```python
from build123d import *

# Parameters (mm, degrees)
SKETCH1_R               = 43
SKETCH1_R_2             = 9.5
SKETCH1_R_3             = 3
BOSS_EXTRUDE1_DEPTH     = 6
CUT_EXTRUDE1_DEPTH      = 62.983868869
CUT_EXTRUDE1_DEPTH_BACK = 62.983868869


with BuildPart() as part:
    # Sketch1 → Boss-Extrude1 (new, symmetric)
    with BuildSketch(Plane(origin=(0, 0, 0), x_dir=(1, 0, 0), z_dir=(0, 1, 0))):
        with Locations(Location((0, 0, 0), (0, 0, 270))):
            Circle(SKETCH1_R)
        with Locations(Location((0, 0, 0), (0, 0, 270))):
            Circle(SKETCH1_R_2, mode=Mode.SUBTRACT)
        with Locations(Location((0, -32, 0), (0, 0, 270))):
            Circle(SKETCH1_R_3, mode=Mode.SUBTRACT)
        with Locations(Location((-30.433808521, -9.88854382, 0), (0, 0, 270))):
            Circle(SKETCH1_R_3, mode=Mode.SUBTRACT)
        with Locations(Location((-18.809128073, 25.88854382, 0), (0, 0, 270))):
            Circle(SKETCH1_R_3, mode=Mode.SUBTRACT)
        with Locations(Location((18.809128073, 25.88854382, 0), (0, 0, 270))):
            Circle(SKETCH1_R_3, mode=Mode.SUBTRACT)
        with Locations(Location((30.433808521, -9.88854382, 0), (0, 0, 270))):
            Circle(SKETCH1_R_3, mode=Mode.SUBTRACT)
    extrude(amount=BOSS_EXTRUDE1_DEPTH, both=True)

    # Sketch2 → Cut-Extrude1 (cut, two sides: drawn at the far end of the back side and taken through both)
    with BuildSketch(Plane(origin=(0, 6, 0), x_dir=(1, 0, 0), z_dir=(0, 1, 0)).offset(-CUT_EXTRUDE1_DEPTH_BACK)):
        with BuildLine():
            ThreePointArc((-9.114016839, 9.270096928), (-12.363734712, 4.017220927), (-12.822220771, -2.142581267))
            ThreePointArc((-12.822220771, -2.142581267), (-21.270303496, -1.833512485), (-29.494654795, 0.122419764))
            ThreePointArc((-29.494654795, 0.122419764), (-32.446074444, 2.845461233), (-32.44271131, 6.861158119))
            ThreePointArc((-32.44271131, 6.861158119), (-31.194730701, 10.135782424), (-30.27959235, 13.518553733))
            ThreePointArc((-30.27959235, 13.518553733), (-27.921945775, 16.769297559), (-23.933633504, 17.23748344))
            ThreePointArc((-23.933633504, 17.23748344), (-16.130325405, 13.985713467), (-9.114016839, 9.270096928))
        make_face()
        with BuildLine():
            ThreePointArc((6, 11.532562595), (0, 13), (-6, 11.532562595))
            ThreePointArc((-6, 11.532562595), (-8.316659253, 19.662674227), (-8.99792146, 28.088913426))
            ThreePointArc((-8.99792146, 28.088913426), (-7.320193957, 31.737346406), (-3.5, 32.975066458))
            ThreePointArc((-3.5, 32.975066458), (0, 32.800080928), (3.5, 32.975066458))
            ThreePointArc((3.5, 32.975066458), (7.320193957, 31.737346406), (8.99792146, 28.088913426))
            ThreePointArc((8.99792146, 28.088913426), (8.316659253, 19.662674227), (6, 11.532562595))
        make_face()
        with BuildLine():
            ThreePointArc((12.822220771, -2.142581267), (12.363734712, 4.017220927), (9.114016839, 9.270096928))
            ThreePointArc((9.114016839, 9.270096928), (16.130325405, 13.985713467), (23.933633504, 17.23748344))
            ThreePointArc((23.933633504, 17.23748344), (27.921945775, 16.769297559), (30.27959235, 13.518553733))
            ThreePointArc((30.27959235, 13.518553733), (31.194730701, 10.135782424), (32.44271131, 6.861158119))
            ThreePointArc((32.44271131, 6.861158119), (32.446074444, 2.845461233), (29.494654795, 0.122419764))
            ThreePointArc((29.494654795, 0.122419764), (21.270303496, -1.833512485), (12.822220771, -2.142581267))
        make_face()
        with BuildLine():
            ThreePointArc((-1.924568248, -12.856750642), (-4.829111259, -20.795847261), (-9.230777689, -28.013253851))
            ThreePointArc((-9.230777689, -28.013253851), (-12.732582852, -29.978754651), (-16.550698277, -28.734637538))
            ThreePointArc((-16.550698277, -28.734637538), (-19.279403843, -26.535822888), (-22.213817238, -24.620140772))
            ThreePointArc((-22.213817238, -24.620140772), (-24.576905478, -21.373350548), (-23.78972044, -17.435562779))
            ThreePointArc((-23.78972044, -17.435562779), (-18.285748603, -11.019027947), (-11.632772181, -5.803327614))
            ThreePointArc((-11.632772181, -5.803327614), (-7.64120828, -10.517220927), (-1.924568248, -12.856750642))
        make_face()
        with BuildLine():
            ThreePointArc((1.924568248, -12.856750642), (7.64120828, -10.517220927), (11.632772181, -5.803327614))
            ThreePointArc((11.632772181, -5.803327614), (18.285748603, -11.019027947), (23.78972044, -17.435562779))
            ThreePointArc((23.78972044, -17.435562779), (24.576905478, -21.373350548), (22.213817238, -24.620140772))
            ThreePointArc((22.213817238, -24.620140772), (19.279403843, -26.535822888), (16.550698277, -28.734637538))
            ThreePointArc((16.550698277, -28.734637538), (12.732582852, -29.978754651), (9.230777689, -28.013253851))
            ThreePointArc((9.230777689, -28.013253851), (4.829111259, -20.795847261), (1.924568248, -12.856750642))
        make_face()
    extrude(amount=CUT_EXTRUDE1_DEPTH + CUT_EXTRUDE1_DEPTH_BACK, mode=Mode.SUBTRACT)


solid = part.part
```
Verification items for the finished model (mm, model axes). Coordinates: 2 decimals unless noted, no trailing zeros. Loops run counter-clockwise (first coordinate to the right, second up) from the corner with the lowest first, then second, coordinate; pieces in that order, holes last. Notation, with made-up numbers: (45.5, 7.25) - (92.5, 7.25) arc R32 cw to (92.5, 39.25) - close; hole circle Ø5 at (42, 84.25). An arc over 180 degrees is marked (long way). Put each result on its own line as item: value.
Item 1: Section check C-C (z = -25). Enter the section's corners in (x, y).
Conclusion:
outline: (-34.99, -6) - (-21.67, -6) - (-21.67, 6) - (-34.99, 6) - close; (-15.94, -6) - (-8.94, -6) - (-8.94, 6) - (-15.94, 6) - close; (8.94, -6) - (15.94, -6) - (15.94, 6) - (8.94, 6) - close; (21.67, -6) - (34.99, -6) - (34.99, 6) - (21.67, 6) - close
Item 2: Gauge pin test, flat ends, axial feed: pin 1 Ø6 at (x, y) = (-5, 0) entering from -Z; pin 2 Ø1.5 at (x, y) = (27.5, 4.5) entering from -Z; pin 3 Ø4 at (y, z) = (1, 18.5) entering from -X. Record the tip position at first contact, or that the pin passes through.
Conclusion:
pin 1: stops at z = -42.95
pin 2: stops at z = -33.67
pin 3: stops at x = -39.71
Item 3: Section check A-A (x = 0). Enter the section's corners in (y, z), then the cut area to 3 significant figures.
Conclusion:
outline: (-6, -43) - (6, -43) - (6, -32.8) - (-6, -32.8) - close; (-6, -13) - (6, -13) - (6, -9.5) - (-6, -9.5) - close; (-6, 9.5) - (6, 9.5) - (6, 29) - (-6, 29) - close; (-6, 35) - (6, 35) - (6, 43) - (-6, 43) - close
area: 494 mm2
Item 4: Scan lines: line 1 along Z through (x, y) = (18, -1.5); line 2 along Z through (x, y) = (29, -0.25); line 3 along X through (y, z) = (1.5, -6.5). Record each from-to range of solid material in increasing order.
Conclusion:
line 1: z = -39.05 to -28.78, -23 to -14.93, 2.15 to 10.75, 27.51 to 39.05
line 2: z = -31.75 to -15.92, 0.04 to 7.25, 12.52 to 31.75
line 3: x = -42.51 to -32.58, -11.26 to -6.93, 6.93 to 11.26, 32.58 to 42.51
Item 5: Draft check along Z on faces 1 (the face through (29.061, 0.084, -31.693)), 2 (the face through (-31.21, -0.08, -10.09)), 3 (the face through (1, -6, -10)), 4 (the face through (0, 0, -13)). Enter one of: pulls with the +Z half, pulls with the -Z half, needs draft (parallel to the pull), parting line crosses it, or undercut.
Conclusion:
face 1: parting line crosses it
face 2: undercut
face 3: needs draft
face 4: undercut
Item 6: Section check B-B (z = 32). Enter the section's corners in (x, y), then the cut area to 3 significant figures.
Conclusion:
outline: (-28.72, -6) - (-3, -6) - (-3, 6) - (-28.72, 6) - close; (3, -6) - (28.72, -6) - (28.72, 6) - (3, 6) - close
area: 617 mm2
Item 7: Section check D-D (z = 21). Enter the section's corners in (x, y).
Conclusion:
outline: (-37.52, -6) - (-24.64, -6) - (-24.64, 6) - (-37.52, 6) - close; (-4.93, -6) - (4.93, -6) - (4.93, 6) - (-4.93, 6) - close; (24.64, -6) - (37.52, -6) - (37.52, 6) - (24.64, 6) - close
